```python
from build123d import *

# Parameters (mm, degrees)
SKETCH1_W                 = 492.125
SKETCH1_H                 = 274.6375
BOSS_EXTRUDE1_DEPTH       = 4.7625
CUT_EXTRUDE1_REACH        = 6.763
BOSS_EXTRUDE2_REACH       = 494.125
SKETCH3_W                 = 4.7625
SKETCH3_H                 = 274.6375
F_8_CLEARANCE_HOLE1_D     = 4.3053
F_8_CLEARANCE_HOLE1_DEPTH = 74.422
F_8_CLEARANCE_HOLE1_TIP   = 1.293442612
SKETCH9_W                 = 381
SKETCH9_H                 = 215.9
CUT_EXTRUDE2_DEPTH        = 5.7625
F_8_CLEARANCE_HOLE2_D     = 4.4958
F_8_CLEARANCE_HOLE2_DEPTH = 74.422
F_8_CLEARANCE_HOLE2_TIP   = 1.350674586
F_6_CLEARANCE_HOLE1_D     = 3.7973
F_6_CLEARANCE_HOLE1_DEPTH = 74.422
F_6_CLEARANCE_HOLE1_TIP   = 1.140824014
SKETCH14_W                = 22.86
SKETCH14_H                = 46.99
CUT_EXTRUDE3_DEPTH        = 46.736


with BuildPart() as part:
    # Sketch1 → Boss-Extrude1 (new body)
    with BuildSketch(Plane(origin=(0, 0, 0), x_dir=(0, 0, -1), z_dir=(1, 0, 0))):
        Rectangle(SKETCH1_W, SKETCH1_H)
    extrude(amount=BOSS_EXTRUDE1_DEPTH)

    # Sketch2 → Cut-Extrude1 (cut, up to next)
    with BuildSketch(Plane(origin=(4.7625, 0, 0), x_dir=(0, 0, -1), z_dir=(1, 0, 0)), mode=Mode.PRIVATE) as cut_extrude1_sk1:
        Polygon((-24.852813742, -60), (24.852813742, -60), (42.426406871, -42.426406871), (60, -24.852813742), (60, 24.852813742), (24.852813742, 60), (-24.852813742, 60), (-60, 24.852813742), (-60, -24.852813742), align=None)
    cut_extrude1_tool1 = extrude(cut_extrude1_sk1.sketch, amount=-CUT_EXTRUDE1_REACH, mode=Mode.PRIVATE) & part.part
    add(cut_extrude1_tool1.solids().sort_by_distance((4.7625, 0, 0))[0], mode=Mode.SUBTRACT)

    # Sketch3 → Boss-Extrude2 (add, up to next)
    with BuildSketch(Plane.XY.offset(246.0625), mode=Mode.PRIVATE) as boss_extrude2_sk1:
        with Locations((2.38125, 0)):
            Rectangle(SKETCH3_W, SKETCH3_H)
    boss_extrude2_tool1 = extrude(boss_extrude2_sk1.sketch, amount=-BOSS_EXTRUDE2_REACH, mode=Mode.PRIVATE) - part.part
    add(boss_extrude2_tool1.solids().sort_by_distance((2.38125, 0, 246.0625))[0])

    # #8 Clearance Hole1
    with Locations(Plane(origin=(4.7625, 0, 0), x_dir=(0, 0, -1), z_dir=(1, 0, 0))):
        with Locations((-231.93375, -98.20275), (-231.93375, -47.40275), (231.93375, -47.40275), (231.93375, -98.20275)):
            Hole(F_8_CLEARANCE_HOLE1_D / 2, depth=F_8_CLEARANCE_HOLE1_DEPTH)
            with Locations((0, 0, -(F_8_CLEARANCE_HOLE1_DEPTH + F_8_CLEARANCE_HOLE1_TIP / 2))):  # 118° drill point
                Cone(0, F_8_CLEARANCE_HOLE1_D / 2, F_8_CLEARANCE_HOLE1_TIP, mode=Mode.SUBTRACT)

    # Sketch9 → Cut-Extrude2 (cut, through all)
    with BuildSketch(Plane(origin=(4.7625, 0, 0), x_dir=(0, 0, -1), z_dir=(1, 0, 0))):
        with Locations((0, -29.36875)):
            Rectangle(SKETCH9_W, SKETCH9_H)
    extrude(amount=-CUT_EXTRUDE2_DEPTH, mode=Mode.SUBTRACT)

    # #8 Clearance Hole2
    with Locations(Plane(origin=(4.7625, 0, 0), x_dir=(0, 0, -1), z_dir=(1, 0, 0))):
        with Locations((-114.3, 88.9), (-84.1375, 88.9), (84.1375, 88.9), (114.3, 88.9)):
            Hole(F_8_CLEARANCE_HOLE2_D / 2, depth=F_8_CLEARANCE_HOLE2_DEPTH)
            with Locations((0, 0, -(F_8_CLEARANCE_HOLE2_DEPTH + F_8_CLEARANCE_HOLE2_TIP / 2))):  # 118° drill point
                Cone(0, F_8_CLEARANCE_HOLE2_D / 2, F_8_CLEARANCE_HOLE2_TIP, mode=Mode.SUBTRACT)

    # #6 Clearance Hole1
    with Locations(Plane(origin=(4.7625, 0, 0), x_dir=(0, 0, -1), z_dir=(1, 0, 0))):
        with Locations((-203.97089, -131.73075), (203.97089, -131.73075)):
            Hole(F_6_CLEARANCE_HOLE1_D / 2, depth=F_6_CLEARANCE_HOLE1_DEPTH)
            with Locations((0, 0, -(F_6_CLEARANCE_HOLE1_DEPTH + F_6_CLEARANCE_HOLE1_TIP / 2))):  # 118° drill point
                Cone(0, F_6_CLEARANCE_HOLE1_D / 2, F_6_CLEARANCE_HOLE1_TIP, mode=Mode.SUBTRACT)

    # Sketch14 → Cut-Extrude3 (cut)
    with BuildSketch(Plane(origin=(4.7625, 0, 0), x_dir=(0, 0, -1), z_dir=(1, 0, 0))):
        with Locations((218.1225, 63.65875)):
            Rectangle(SKETCH14_W, SKETCH14_H)
    extrude(amount=-CUT_EXTRUDE3_DEPTH, mode=Mode.SUBTRACT)


solid = part.part
```
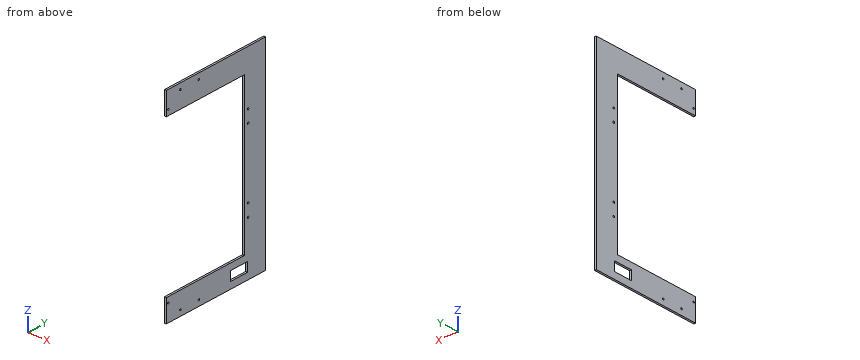
Can you work these out from the model? Positions are in its coordinate system, mm. Give positions to 0.01 mm unless a question says otherwise; leave off trailing zeros. Loops run counter-clockwise (first coordinate to the right, second up) from the corner with the lowest first, then second, coordinate; pieces in that order, holes last. Notation, with made-up numbers: M 58,58.25 L 116,58.25 A15 ccw 116,65.25 Z; hole C -17,5 d2. An arc over 180 degrees is marked long. Use one line per item in the form item = value. Start each with the question number.
(1) I'm going to push a flat-ended pin straight in: P1, Ø1.5, axis at x = 3.5, z = -111, coming from the -Y side. Where does the tip first touch, or does it pass through?
(2) Please list where these lines run through material, in increasing order: line 1 (Z direction, x = 3.1, y = -34.5); line 2 (Y direction, x = 1.65, z = 18.5); line 3 (Y direction, x = 3.3, z = -219).
(3) I want a section at A-A, the plane y = 21.5. Write out the boundary of the cut face in (x, z).
(4) I want a section at B-B, the plane x = 2.4. State how many separate pieces and enclosed holes the cut face has, and give its area (3 significant figures).
(5) I want a section at C-C, the plane z = 53. Write out the boundary of the cut face in (x, y), and give its area (3 significant figures).
Worked out:
q1.P1 = 78.58
q2.line_1 = -246.06 to -190.5, 190.5 to 246.06
q2.line_2 = 78.58 to 137.32
q2.line_3 = -137.32 to 40.16, 87.15 to 137.32
q3.outline = M 0,-246.06 L 4.76,-246.06 L 4.76,-190.5 L 0,-190.5 Z; M 0,190.5 L 4.76,190.5 L 4.76,246.06 L 0,246.06 Z
q4.separate_pieces = 1
q4.enclosed_holes = 11
q4.area = 51,700 mm²
q5.outline = M 0,78.58 L 4.76,78.58 L 4.76,137.32 L 0,137.32 Z
q5.area = 280 mm²
